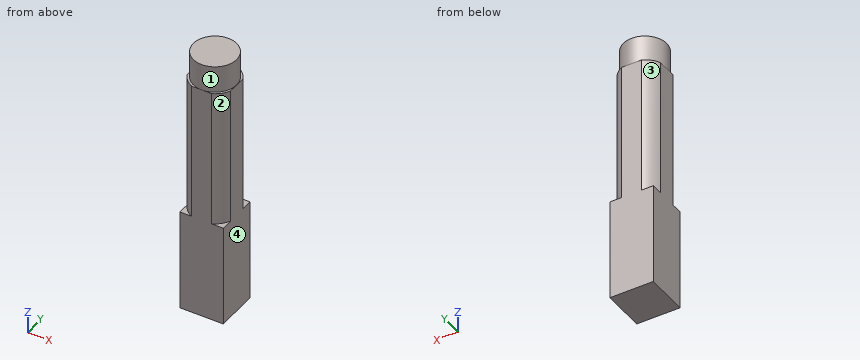
from build123d import *

# Parameters (mm, degrees)
SKETCH1_W           = 6.35
SKETCH1_H           = 6.35
BOSS_EXTRUDE1_DEPTH = 39.37
SKETCH2_W           = 6.35
SKETCH2_H           = 6.35
SKETCH2_R           = 3.17373
CUT_EXTRUDE1_DEPTH  = 3.96875
SKETCH3_W           = 9.525
SKETCH3_H           = 9.525
SKETCH3_R           = 3.4925
CUT_EXTRUDE2_DEPTH  = 20.394676


with BuildPart() as part:
    # Sketch1 → Boss-Extrude1 (new body)
    with BuildSketch(Plane.XY):
        Rectangle(SKETCH1_W, SKETCH1_H)
    extrude(amount=BOSS_EXTRUDE1_DEPTH)

    # Sketch2 → Cut-Extrude1 (cut)
    with BuildSketch(Plane.XY.offset(39.37)):
        Rectangle(SKETCH2_W, SKETCH2_H)
        Circle(SKETCH2_R, mode=Mode.SUBTRACT)
    extrude(amount=-CUT_EXTRUDE1_DEPTH, mode=Mode.SUBTRACT)

    # Sketch3 → Cut-Extrude2 (cut)
    with BuildSketch(Plane.XY.offset(35.40125)):
        Rectangle(SKETCH3_W, SKETCH3_H)
        Circle(SKETCH3_R, mode=Mode.SUBTRACT)
    extrude(amount=-CUT_EXTRUDE2_DEPTH, mode=Mode.SUBTRACT)


solid = part.part
Build history of the part. All positions in model axes, mm. Face numbers are marked on the shaded views. A direction names the side the tool comes from. Round coordinates to 2 decimals unless told otherwise and drop trailing zeros. Loops run counter-clockwise (first coordinate to the right, second up) from the corner with the lowest first, then second, coordinate; pieces in that order, holes last. Notation, with made-up numbers: (42.5, 64) -> (72.5, 64) arc R18 cw to (72.5, 70) -> close; hole circle Ø4 at (-2, 60.5). An arc over 180 degrees is marked (long way). One line per item, written item: value. Start each with the question number.
Q1. Probe line 1 along Y through (x, z) = (0, 38.5); line 2 along Z through (x, y) = (2.5, 2); line 3 along X through (y, z) = (-1.75, 18.5). List the from-to ranges inside material, lowest first.
Q2. Cut at A-A on z = 28.5. List the corners of the cut face in (x, y) (1 decimal), plus the area to 3 significant figures.
Q3. 3-axis set-ups, long thin cutter, end or side, ignore diameter. For the marked faces 1, 2, 3 and 4: which of +Z, -Z, +X, -X, +Y, -Y reach the whole face in a straight line?
Q4. Drop flat-ended pins along their axis: pin 1 Ø1.9 at (x, y) = (-2, 2.5) entering from +Z; pin 2 Ø1 at (x, z) = (-2, 28) entering from +Y. Give the stop position or say it passes through.
Computed:
1. line 1: -3.17 to 3.17
1. line 2: 0 to 35.4
1. line 3: -3.02 to 3.02
2. outline: (-3.2, -1.5) arc R3.5 ccw to (-1.5, -3.2) -> (1.5, -3.2) arc R3.5 ccw to (3.2, -1.5) -> (3.2, 1.5) arc R3.5 ccw to (1.5, 3.2) -> (-1.5, 3.2) arc R3.5 ccw to (-3.2, 1.5) -> close
2. area: 35.8 mm²
3. face 1: +Z
3. face 2: +Z, +X, -Y
3. face 3: +Z, -X, +Y
3. face 4: +Z, -Z, +X, +Y, -Y
4. pin 1: z = 39.37
4. pin 2: y = 3.15
